The figure shows three views and two pictorial views of one solid part (mm, origin at its lowest corner). Answer the questions. A direction names the side the tool comes from. Give positions to 0.01 mm unless a question says otherwise; leave off trailing zeros. Order: outer loops, then holes, each group sorted by start corner. A loop starts at its lowest first (then second) coordinate and runs counter-clockwise, first axis right, second up. Notation, with made-up numbers: (55.5, 22.5) - (94.5, 22.5) arc R8 cw to (94.5, 34.5) - close; hole circle Ø8 at (-16, -23). An arc over 180 degrees is marked (long way). Use a Markdown table: item, result. Add a question column.
1. A cutting plane is placed at B-B on y = 19.5. Determine the outline of the cut face in (x, z).
2. A cutting plane is placed at D-D on z = 57.5. Determine the outline of the cut face in (x, y).
3. A cutting plane is placed at C-C on x = 58. Determine the outline of the cut face in (y, z).
4. Flat-ended cylindrical pins translate along their axes: P1, Ø1, axis at x = 75, z = 64.5, coming from the -Y side; P2, Ø2.5, axis at x = 1.5, z = 28.5, coming from the +Y side; P3, Ø2, axis at y = 135, z = 47.5, coming from the -X side; P4, Ø17.5, axis at x = 102.37, z = 70, coming from the -Y side. Find the tip coordinate at first contact, or state that the pin passes through.
5. A cutting plane is placed at A-A on z = 46. Determine the outline of the cut face in (x, y).
6. For a pull along X with two mould halves and no side action, classify the marked faces 3, 4, 5 and 6 as released by +X, released by -X, zero draft, split by the parting line, or undercut.
7. Consider L1, parallel to X at y = 28.5, z = 60; L2, parallel to X at y = 40.5, z = 32; L3, parallel to Y at x = 170, z = 8. Determine where each line is inside the solid, lowest interval first.
8. Which of the six approach directions +Z, -Z, +X, -X, +Y, -Y give full straight-line access (tool end or side, diameter ignored) to the marked faces 1 and 2?
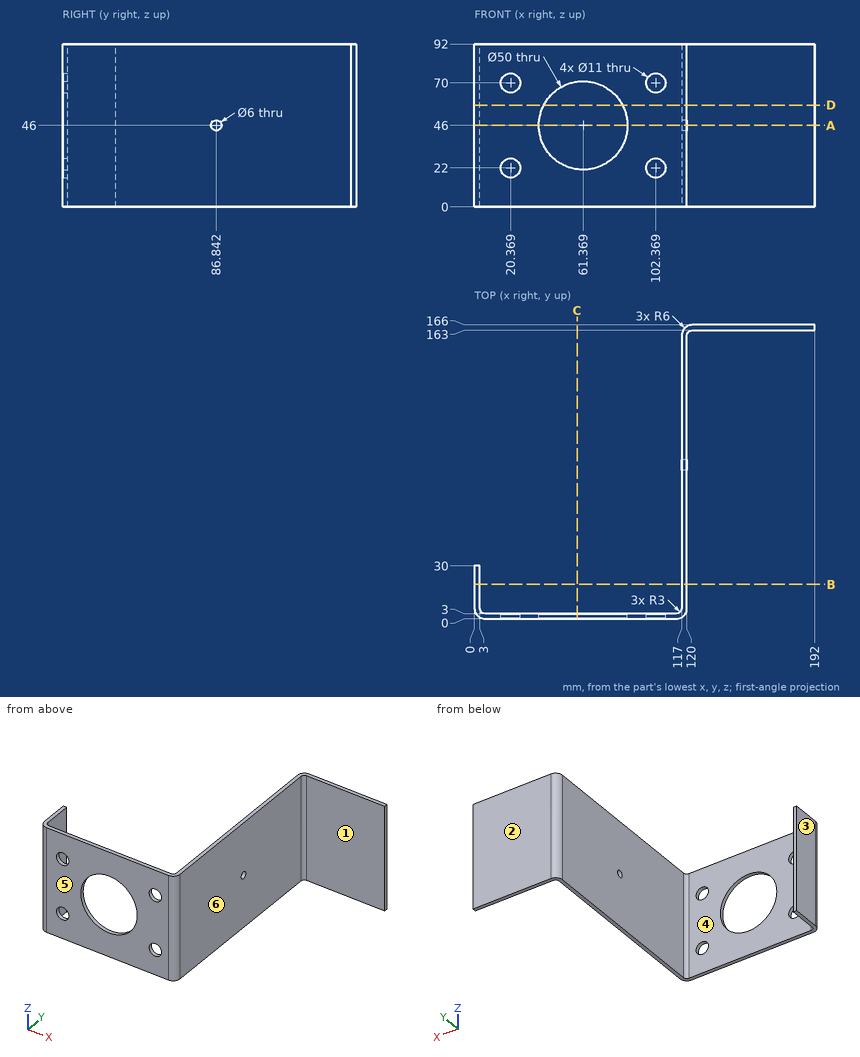
Output values:
| question | item | result |
|---|---|---|
| 1 | outline | (0, 0) - (3, 0) - (3, 92) - (0, 92) - close; (117, 0) - (120, 0) - (120, 92) - (117, 92) - close |
| 2 | outline | (0, 6) arc R6 ccw to (6, 0) - (39.17, 0) - (39.17, 3) - (6, 3) arc R3 cw to (3, 6) - (3, 30) - (0, 30) - close; (83.57, 0) - (114, 0) arc R6 ccw to (120, 6) - (120, 160) arc R3 cw to (123, 163) - (192, 163) - (192, 166) - (123, 166) arc R6 ccw to (117, 160) - (117, 6) arc R3 cw to (114, 3) - (83.57, 3) - close |
| 3 | outline | (0, 0) - (3, 0) - (3, 21.23) - (0, 21.23) - close; (0, 70.77) - (3, 70.77) - (3, 92) - (0, 92) - close |
| 4 | P1 | through |
| 4 | P2 | y = 30 |
| 4 | P3 | x = 117 |
| 4 | P4 | y = 0 |
| 5 | outline | (0, 6) arc R6 ccw to (6, 0) - (36.37, 0) - (36.37, 3) - (6, 3) arc R3 cw to (3, 6) - (3, 30) - (0, 30) - close; (86.37, 0) - (114, 0) arc R6 ccw to (120, 6) - (120, 83.84) - (117, 83.84) - (117, 6) arc R3 cw to (114, 3) - (86.37, 3) - close; (117, 89.84) - (120, 89.84) - (120, 160) arc R3 cw to (123, 163) - (192, 163) - (192, 166) - (123, 166) arc R6 ccw to (117, 160) - close |
| 6 | face 3 | released by -X |
| 6 | face 4 | undercut |
| 6 | face 5 | zero draft |
| 6 | face 6 | released by +X |
| 7 | L1 | 0 to 3, 117 to 120 |
| 7 | L2 | 117 to 120 |
| 7 | L3 | 163 to 166 |
| 8 | face 1 | +Z, -Z, +X, -Y |
| 8 | face 2 | +Z, -Z, +X, -X, +Y |
